Read the model definition and answer for the solid it produces. Units are mm, in the model's axes. Face numbers are marked on the shaded views. A direction names the side the tool comes from. Coordinates: 2 decimals unless noted, no trailing zeros. Write each loop counter-clockwise with the first axis right and the second up, starting at its lowest first coordinate (ties: lowest second). Pieces come first, ordered by that corner, then holes.
(1) Given pin 1 (12 mm diameter, centred on y = 11, z = -18, fed in from +X); pin 2 (5 mm diameter, centred on x = 6.5, z = -7.5, fed in from +Y); pin 3 (10 mm diameter, centred on y = 15, z = 20.2, fed in from +X); pin 4 (12 mm diameter, centred on y = 7.5, z = 23.5, fed in from +X), each flat-ended and moving along its own axis, determine where each tip first touches the part or whether it passes through.
(2) Section C-C on z = 20.2 is taken. Write down the section's boundary in (x, y) (3 decimals), then the cut area to 3 significant figures.
(3) Section B-B on y = 15 is taken. State how many separate pieces and enclosed holes the cut face has, then the cut area to 3 significant figures.
(4) Which of the six approach directions +Z, -Z, +X, -X, +Y, -Y give full straight-line access (tool end or side, diameter ignored) to the marked faces 5 and 6?
(5) Section D-D on x = 10.5 is taken. Write down the section's boundary in (y, z), then the cut area to 3 significant figures.
(6) The mould has two halves that part along Z. Classify the marked faces 1, 2, 3 and 4: +Z half, -Z half, draft (parallel to the pull), parting line (faces both ways), or undercut.
(7) Section A-A on x = 2.75 is taken. Write down the section's boundary in (y, z) (3 decimals).
(8) Find the intervals of material crossed by probe 1 along Y at (x, z) = (4.05, -20.2) (3 decimals); probe 2 along Y at (x, z) = (3, -21); probe 3 along X at (y, z) = (6.75, -24.5), in increasing order.
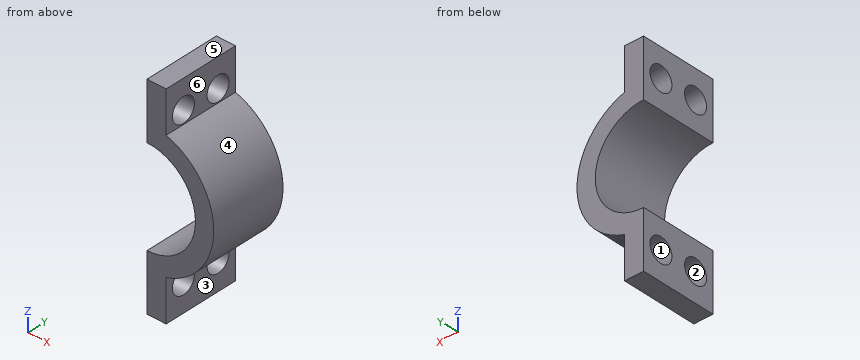
Autodesk Inventor part; units mm, degrees
ref_plane "YZ Plane" through (0, 0, 0) normal (1, 0, 0) x (0, 1, 0)
ref_plane "XZ Plane" through (0, 0, 0) normal (0, 1, 0) x (-1, 0, 0)
ref_plane "XY Plane" through (0, 0, 0) normal (0, 0, 1) x (1, 0, 0)
sketch "Sketch1" plane through (0, 0, 0) normal (0, 1, 0) x (-1, 0, 0)
  circle A0 centre (0, 0) radius 12.7
  circle A1 centre (0, 0) radius 17.5
  dimension "d0" = 25.4
  dimension "d1" = 35
extrude "Extrusion1" add sketch "Sketch1" along normal blind 20
sketch "Sketch2" plane through (0, 20, 0) normal (0, 1, 0) x (1, 0, 0)
  circle A0 centre (0, 0) radius 17.5
  line L0 (0, -17.5) -> (-17.5, -17.5)
  line L1 (-17.5, -17.5) -> (-17.5, 18.3836)
  line L2 (-17.5, 18.3836) -> (0, 18.3836)
  line L3 (0, 18.3836) -> (0, -17.5)
extrude "Extrusion2" cut sketch "Sketch2" against normal blind 20 contours L0 L1 A0 | A0 L3 | L1 L2 L3 A0 picked at (-8.2181, -1.8757)
sketch "Sketch3" plane through (0, 20, 12.7) normal (-1, 0, 0) x (0, 0, 1)
  line L0 (-25.4, 0) -> (-25.4, -20)
  line L1 (-25.4, -20) -> (-40.4, -20)
  line L2 (-40.4, -20) -> (-40.4, 0)
  line L3 (-40.4, 0) -> (-25.4, 0)
  line L4 (-25.4, 0) -> (-25.4, -20)
  line L5 (-25.4, 0) -> (0, 0)
  line L6 (0, 0) -> (15, 0)
  line L7 (15, 0) -> (15, -20)
  line L8 (15, -20) -> (0, -20)
  line L9 (0, -20) -> (0, 0)
  point P0 (-12.7, -20)
  dimension "d6" = 15
  dimension "d7" = 15
sketch "Sketch4" plane through (0, 20, 12.7) normal (-1, 0, 0) x (0, 0, 1)
  line L0 (-25.4, 0) -> (-25.4, -20) construction
  line L1 (-25.4, -10) -> (-40.4302, -10) construction
  line L2 (-40.4302, -10) -> (15.0302, -10) construction
  point P0 (-12.7, -20)
extrude "Extrusion3" add sketch "Sketch3" against normal blind 5
sketch "Sketch5" plane through (0, 0, 12.7) normal (-1, 0, 0) x (0, 0, 1)
  line L0 (-29.4705, 0) -> (-40.4, 0) construction
  line L1 (-40.4, 0) -> (-25.4, 10) construction
  line L2 (-25.4, 20) -> (-25.4, 0) construction
  line L3 (-40.4, 10) -> (-25.4, 0) construction
  line L4 (-25.4, 0) -> (-40.4, 10) construction
  line L5 (-25.4, 20) -> (0, 20) construction
  line L6 (-40.4, 10) -> (-25.4, 20) construction
  line L7 (-25.4, 20) -> (-40.4, 20) construction
  line L8 (-40.4, 20) -> (-25.4, 10) construction
  line L9 (0, 0) -> (-25.4, 0) construction
  line L10 (0, 0) -> (15, 10) construction
  line L11 (15, 20) -> (15, 0) construction
  line L12 (0, 0) -> (0, 20) construction
  line L13 (0, 10) -> (15, 0) construction
  line L14 (0, 10) -> (15, 20) construction
  line L15 (0, 20) -> (15, 10) construction
  circle A0 centre (-32.9, 15) radius 3.175 construction
  circle A1 centre (-32.9, 15) radius 3.175
  circle A2 centre (-32.9, 5) radius 3.175
  circle A3 centre (7.5, 5) radius 3.175
  circle A4 centre (7.5, 15) radius 3.175
  point P0 (-12.7, 0)
  dimension "d10" = 6.35
  dimension "d11" = 6.35
  dimension "d12" = 6.35
  dimension "d13" = 6.35
  dimension "d14" = 6.35
extrude "Extrusion4" cut sketch "Sketch5" against normal blind 5
properties part number "scopeCupler"
Response:
1. pin 1: stops at x = 12.74
1. pin 2: passes through
1. pin 3: stops at x = 8.67
1. pin 4: stops at x = 5
2. outline: (0, 0) - (5, 0) - (5, 1.825) - (0, 1.825) - close; (0, 8.175) - (5, 8.175) - (5, 11.825) - (0, 11.825) - close; (0, 18.175) - (5, 18.175) - (5, 20) - (0, 20) - close
2. area: 36.5 mm2
3. separate pieces: 3
3. enclosed holes: 0
3. area: 269 mm2
4. face 5: +Z, +X, -X, +Y, -Y
4. face 6: +Z, +X, +Y, -Y
5. outline: (0, -14) - (20, -14) - (20, -7.14) - (0, -7.14) - close; (0, 7.14) - (20, 7.14) - (20, 14) - (0, 14) - close
5. area: 274 mm2
6. face 1: undercut
6. face 2: undercut
6. face 3: draft
6. face 4: parting line
7. outline: (0, -27.7) - (20, -27.7) - (20, -12.399) - (0, -12.399) - close; (0, 12.399) - (20, 12.399) - (20, 27.7) - (0, 27.7) - close; hole circle Ø6.35 at (5, -20.2); hole circle Ø6.35 at (5, 20.2); hole circle Ø6.35 at (15, -20.2); hole circle Ø6.35 at (15, 20.2)
8. probe 1: y = 0 to 1.825, 8.175 to 11.825, 18.175 to 20
8. probe 2: y = 0 to 1.93, 8.07 to 11.93, 18.07 to 20
8. probe 3: x = 0 to 5
